The model under review builds one solid part; all positions refer to its coordinate system, in mm. A direction names the side the tool comes from. Give positions to 0.01 mm unless a question says otherwise; leave off trailing zeros. Loops run counter-clockwise (first coordinate to the right, second up) from the corner with the lowest first, then second, coordinate; pieces in that order, holes last. Notation, with made-up numbers: (0, 38.5) - (26, 38.5) arc R15 cw to (26, 67.5) - close; hole circle Ø5 at (51.5, -24.5). An arc over 180 degrees is marked (long way). Answer as a JSON object with one key per item and string values.
from build123d import *

# Parameters (mm, degrees)
F0_W     = 50.8
F0_H     = 76.2
F1_DEPTH = 50.8
F2_R     = 12.7
F3_DEPTH = 25.4
F4_W     = 38.1
F4_H     = 25.4
F5_DEPTH = 2.54


with BuildPart() as f1:
    # F0 (on Top) → F1 (new body)
    with BuildSketch(Plane.XY):
        Rectangle(F0_W, F0_H)
    extrude(amount=F1_DEPTH)

    # F2 (on face) → F3 (cut)
    with BuildSketch(Plane.XY.offset(50.8)):
        Circle(F2_R)
    extrude(amount=-F3_DEPTH, mode=Mode.SUBTRACT)

    # F4 (on face) → F5 (cut)
    with BuildSketch(Plane.YZ.offset(25.4)):
        with Locations((-19.05, 12.7)):
            Rectangle(F4_W, F4_H)
    extrude(amount=-F5_DEPTH, mode=Mode.SUBTRACT)


solid = f1.part
Q1. Consider section D-D, the plane y = -5. State the section outline as (x, z) points.
Results:
{"outline": "(-25.4, 0) - (22.86, 0) - (22.86, 25.4) - (25.4, 25.4) - (25.4, 50.8) - (11.67, 50.8) - (11.67, 25.4) - (-11.67, 25.4) - (-11.67, 50.8) - (-25.4, 50.8) - close"}
Q2. Consider section C-C, the plane z = 42.5. State the section outline as (x, y) points.
Results:
{"outline": "(-25.4, -38.1) - (25.4, -38.1) - (25.4, 38.1) - (-25.4, 38.1) - close; hole circle Ø25.4 at (0, 0)"}
Q3. To check wall thickness, follow probe 1 along Y at (x, z) = (0, 35); probe 2 along X at (y, z) = (2, 47); probe 3 along Z at (x, y) = (3, 5). State the ranges of each line that lie inside material, in increasing order. Write a range as [from, to].
Results:
{"probe 1": "y = [-38.1, -12.7], [12.7, 38.1]", "probe 2": "x = [-25.4, -12.54], [12.54, 25.4]", "probe 3": "z = [0, 25.4]"}
Q4. Clearance check with flat-ended pins moving along their axes: pin 1 Ø1.3 at (x, y) = (24.5, -10) entering from -Z; pin 2 Ø1.3 at (x, z) = (24, 14) entering from -Y; pin 3 Ø20.5 at (y, z) = (-25, 9) entering from +X. State where each tip first meets the part, or that it passes through.
Results:
{"pin 1": "stops at z = 25.4", "pin 2": "stops at y = 0", "pin 3": "stops at x = 22.86"}
Q5. The part is to be moulded in two halves that separate along Y. For faces 4 (the face through (0, -38.1, 25)), 5 (the face through (-2.75, -12.4, 38.28)), 6 (the face through (22.86, -19, 13)), say which applies: +Y half, -Y half, draft (parallel to the pull), parting line (faces both ways), or undercut.
Results:
{"face 4": "-Y half", "face 5": "undercut", "face 6": "draft"}
Q6. Consider section A-A, the plane x = 0. State the section outline as (y, z) points.
Results:
{"outline": "(-38.1, 0) - (38.1, 0) - (38.1, 50.8) - (12.7, 50.8) - (12.7, 25.4) - (-12.7, 25.4) - (-12.7, 50.8) - (-38.1, 50.8) - close"}
Q7. For faces 1 (the face through (0, 0, 25.4)), 2 (the face through (-25.4, -1, 25)), 3 (the face through (24, -19, 25.4)), list the 3-axis set-ups (+Z, -Z, +X, -X, +Y, -Y) from which the entire face can be reached by the end or side of a thin tool; tool diameter is ignored.
Results:
{"face 1": "+Z", "face 2": "+Z, -Z, -X, +Y, -Y", "face 3": "-Z, +X, -Y"}
Q8. Consider section B-B, the plane z = 15. State the section outline as (x, y) points, plus the area to 3 significant figures.
Results:
{"outline": "(-25.4, -38.1) - (22.86, -38.1) - (22.86, 0) - (25.4, 0) - (25.4, 38.1) - (-25.4, 38.1) - close", "area": "3,770 mm^2"}
